```python
from build123d import *

# Parameters (mm, degrees)
SKETCH1_R                                        = 1.27
BOSS_EXTRUDE1_DEPTH                              = 25.4
CSK_FOR_1_4_FLAT_HEAD_MACHINE_SCREW1_D           = 6.7564
CSK_FOR_1_4_FLAT_HEAD_MACHINE_SCREW1_CSINK_D     = 13.3194044
CSK_FOR_1_4_FLAT_HEAD_MACHINE_SCREW1_CSINK_ANGLE = 82
SKETCH4_R                                        = 1.016
CUT_EXTRUDE1_DEPTH                               = 40.37
SKETCH5_W                                        = 65.738203623
SKETCH5_H                                        = 8.173238607
CUT_EXTRUDE2_DEPTH                               = 40.37
FILLET1_R                                        = 0.762
SKETCH8_W                                        = 13.691843982
SKETCH8_H                                        = 25.635792988
SKETCH8_W_2                                      = 17.381844488
SKETCH8_H_2                                      = 26.703951029
CUT_EXTRUDE3_DEPTH                               = 22.082
SKETCH9_R                                        = 5.08
CUT_EXTRUDE4_DEPTH                               = 11.557
CHAMFER1_SIZE                                    = 0.762
SKETCH10_W                                       = 31.402844339
SKETCH10_H                                       = 33.249058222
SKETCH10_W_2                                     = 26.204679654
SKETCH10_H_2                                     = 29.468553059
CUT_EXTRUDE5_DEPTH                               = 2.54
SKETCH11_W                                       = 51.569967854
SKETCH11_H                                       = 49.340439169
CUT_EXTRUDE6_DEPTH                               = 22.082
FILLET3_R                                        = 2.54


with BuildPart() as part:
    # Sketch1 → Boss-Extrude1 (new body)
    with BuildSketch(Plane.XY):
        Polygon((-5.842, 18.669), (-5.842, -1.651), (-28.575, -1.651), (-28.575, -20.701), (28.575, -20.701), (28.575, -1.651), (5.842, -1.651), (5.842, 18.669), align=None)
        with Locations((14.2875, -11.176)):
            Circle(SKETCH1_R, mode=Mode.SUBTRACT)
        with Locations((-14.2875, -11.176)):
            Circle(SKETCH1_R, mode=Mode.SUBTRACT)
    extrude(amount=BOSS_EXTRUDE1_DEPTH)

    # CSK for 1/4 Flat Head Machine Screw1 (through all)
    with Locations(Plane.XY.offset(25.4)):
        with Locations((-14.2875, -11.176), (14.2875, -11.176)):
            CounterSinkHole(CSK_FOR_1_4_FLAT_HEAD_MACHINE_SCREW1_D / 2, CSK_FOR_1_4_FLAT_HEAD_MACHINE_SCREW1_CSINK_D / 2, counter_sink_angle=CSK_FOR_1_4_FLAT_HEAD_MACHINE_SCREW1_CSINK_ANGLE)

    # Sketch4 → Cut-Extrude1 (cut, through all)
    with BuildSketch(Plane(origin=(0, 18.669, 0), x_dir=(1, 0, 0), z_dir=(0, 1, 0))):
        with Locations(Location((0, -5.334, 0), (0, 0, 270))):  # turned: the seam where the file's is
            Circle(SKETCH4_R)
        with Locations(Location((0, -15.494, 0), (0, 0, 90))):  # turned: the seam where the file's is
            Circle(SKETCH4_R)
    extrude(amount=-CUT_EXTRUDE1_DEPTH, mode=Mode.SUBTRACT)

    # Sketch5 → Cut-Extrude2 (cut, through all)
    with BuildSketch(Plane(origin=(0, 18.669, 0), x_dir=(1, 0, 0), z_dir=(0, 1, 0))):
        with Locations((0.634161588, -25.168619304)):
            Rectangle(SKETCH5_W, SKETCH5_H)
    extrude(amount=-CUT_EXTRUDE2_DEPTH, mode=Mode.SUBTRACT)

    # Fillet1
    fillet1_edges = [part.edges().sort_by_distance(p)[0] for p in [
        (-5.842, 18.669, 10.541),
        (5.842, 18.669, 10.541),
    ]]
    fillet(fillet1_edges, radius=FILLET1_R)

    # Sketch8 → Cut-Extrude3 (cut, through all)
    with BuildSketch(Plane.XY.offset(21.082)):
        with Locations((30.340921991, -12.055237245)):
            Rectangle(SKETCH8_W, SKETCH8_H)
        with Locations((-32.185922244, -9.773263248)):
            Rectangle(SKETCH8_W_2, SKETCH8_H_2)
    extrude(amount=-CUT_EXTRUDE3_DEPTH, mode=Mode.SUBTRACT)

    # Sketch9 → Cut-Extrude4 (cut)
    with BuildSketch(Plane.XY.offset(21.082)):
        with Locations((14.2875, -11.176)):
            Circle(SKETCH9_R)
        with Locations((-14.2875, -11.176)):
            Circle(SKETCH9_R)
    extrude(amount=-CUT_EXTRUDE4_DEPTH, mode=Mode.SUBTRACT)

    # Chamfer1
    chamfer1_edges = [part.edges().sort_by_distance(p)[0] for p in [
        (9.2075, -11.176, 21.082),
        (-19.3675, -11.176, 21.082),
        (0, -20.701, 4.318),
        (0, -20.701, 16.51),
    ]]
    chamfer(chamfer1_edges, length=CHAMFER1_SIZE)

    # Sketch10 → Cut-Extrude5 (cut)
    with BuildSketch(Plane(origin=(0, -1.651, 0), x_dir=(1, 0, 0), z_dir=(0, 1, 0))):
        with Locations((-21.54342217, -13.037102767)):
            Rectangle(SKETCH10_W, SKETCH10_H)
        with Locations((18.944339827, -12.019274454)):
            Rectangle(SKETCH10_W_2, SKETCH10_H_2)
    extrude(amount=-CUT_EXTRUDE5_DEPTH, mode=Mode.SUBTRACT)

    # Sketch11 → Cut-Extrude6 (cut, through all)
    with BuildSketch(Plane.XY.offset(21.082)):
        with Locations((0.48369004, -1.756987777)):
            Rectangle(SKETCH11_W, SKETCH11_H)
        with BuildLine():
            Line((14.2875, -4.191), (5.842, -4.191))
            Line((5.842, -4.191), (5.842, 17.907))
            ThreePointArc((5.842, 17.907), (5.618815367, 18.445815367), (5.08, 18.669))
            Line((5.08, 18.669), (-5.08, 18.669))
            ThreePointArc((-5.08, 18.669), (-5.618815367, 18.445815367), (-5.842, 17.907))
            Line((-5.842, 17.907), (-5.842, -4.191))
            Line((-5.842, -4.191), (-14.2875, -4.191))
            ThreePointArc((-14.2875, -4.191), (-21.2725, -11.176), (-14.2875, -18.161))
            Line((-14.2875, -18.161), (14.2875, -18.161))
            ThreePointArc((14.2875, -18.161), (21.2725, -11.176), (14.2875, -4.191))
        make_face(mode=Mode.SUBTRACT)
    extrude(amount=-CUT_EXTRUDE6_DEPTH, mode=Mode.SUBTRACT)

    # Fillet3
    fillet3_edges = [part.edges().sort_by_distance(p)[0] for p in [
        (-5.842, -4.191, 10.541),
        (5.842, -4.191, 10.541),
    ]]
    fillet(fillet3_edges, radius=FILLET3_R)


solid = part.part
```
Could you check a few things on this model? Use its own coordinates, in mm. A direction names the side the tool comes from. Round coordinates to 2 decimals unless told otherwise and drop trailing zeros. Write each loop counter-clockwise with the first axis right and the second up, starting at its lowest first coordinate (ties: lowest second). Pieces come first, ordered by that corner, then holes. Notation, with made-up numbers: M 12,84.5 L 38,84.5 A21 cw 38,105.5 Z; hole C 82,29 d11. An arc over 180 degrees is marked long. Answer in a Markdown table with one row per item. Add a question column.
Q1. On a 3-axis mill with a long thin cutter (end or side, diameter ignored), from which of +Z, -Z, +X, -X, +Y, -Y can I reach the whole of each face in a straight line? I mean faces 5 (the cylindrical face through (13.186, -16.135, 14.998)), 6 (the flat face through (-11, -4.191, 10)), 7 (the flat face through (5.842, 8, 10)), 8 (the cylindrical face through (-0.04, 0.51, 16.51)). Say none if no direction works.
Q2. Imagine slicing it at C-C (z = 5.75). Please give me the cut outline in (x, y) (1 decimal), then the cut area to 3 significant figures.
Q3. If I drill on line 1 (X direction, y = -13, z = 8); line 2 (X direction, y = -10, z = 6); line 3 (X direction, y = -15.5, z = 18), over which ranges is the centre line in solid material (lowest first)? Write a range as from..to.
Q4. Imagine slicing it at A-A (z = 16). Please give me the cut outline in (x, y) (1 decimal), then the cut area to 3 significant figures.
Q5. If we mould it in two halves opening along X, with no side actions, what happens to faces 1 (the cylindrical face through (0.31, 0.51, 6.3)), 2 (the cylindrical face through (6.57, -3.43, 10.39)), 3 (the cylindrical face through (17.662, -11.027, 4.696)), 4 (the cylindrical face through (-6.61, -3.47, 10.39))? For each: +X half, -X half, draft (parallel to the pull), parting line (faces both ways), or undercut.
Q6. Imagine slicing it at B-B (x = 0). Please give me the cut outline in (y, z), then the cut area to 3 significant figures.
Q7. Will these pins go through, and if not, where does the flat tip stop? pin 1 Ø6.5 at (x, z) = (-12, 14.5) entering from +Y; pin 2 Ø2 at (y, z) = (10, 8.5) entering from -X; pin 3 Ø3 at (y, z) = (-4, 17) entering from +X; pin 4 Ø1.5 at (x, y) = (-5, -8) entering from -Z.
Q8. Imagine slicing it at D-D (y = 10). Please give me the cut outline in (x, z).
Values:
| question | item | result |
|---|---|---|
| 1 | face 5 | +Z |
| 1 | face 6 | +Z, -Z, -X, +Y |
| 1 | face 7 | +Z, -Z, +X, +Y |
| 1 | face 8 | +Y, -Y |
| 2 | outline | M -14.3,-18.2 L -0.9,-18.2 L -0.9,18.7 L -5.1,18.7 A0.8 ccw -5.8,17.9 L -5.8,-1.7 A2.5 cw -8.4,-4.2 L -14.3,-4.2 A7 ccw Z; M 0.9,-18.2 L 14.3,-18.2 A7 ccw 14.3,-4.2 L 8.4,-4.2 A2.5 cw 5.8,-1.7 L 5.8,17.9 A0.8 ccw 5.1,18.7 L 0.9,18.7 Z; hole C -14.3,-11.2 d6.8; hole C 14.3,-11.2 d6.8 |
| 2 | area | 682 mm^2 |
| 3 | line 1 | -21.03..-17.13, -11.44..11.44, 17.13..21.03 |
| 3 | line 2 | -21.17..-17.45, -11.12..-0.77, 0.77..11.12, 17.45..21.17 |
| 3 | line 3 | -19.77..-16.95, -11.62..11.62, 16.95..19.77 |
| 4 | outline | M -14.3,-18.2 L -0.9,-18.2 L -0.9,18.7 L -5.1,18.7 A0.8 ccw -5.8,17.9 L -5.8,-1.7 A2.5 cw -8.4,-4.2 L -14.3,-4.2 A7 ccw Z; M 0.9,-18.2 L 14.3,-18.2 A7 ccw 14.3,-4.2 L 8.4,-4.2 A2.5 cw 5.8,-1.7 L 5.8,17.9 A0.8 ccw 5.1,18.7 L 0.9,18.7 Z; hole C -14.3,-11.2 d10.2; hole C 14.3,-11.2 d10.2 |
| 4 | area | 595 mm^2 |
| 5 | face 1 | undercut |
| 5 | face 2 | +X half |
| 5 | face 3 | undercut |
| 5 | face 4 | -X half |
| 6 | outline | M -18.16,0 L 18.67,0 L 18.67,4.32 L -18.16,4.32 Z; M -18.16,6.35 L 18.67,6.35 L 18.67,14.48 L -18.16,14.48 Z; M -18.16,16.51 L 18.67,16.51 L 18.67,21.08 L -18.16,21.08 Z |
| 6 | area | 627 mm^2 |
| 7 | pin 1 | y = -4.19 |
| 7 | pin 2 | x = -5.84 |
| 7 | pin 3 | x = 18.36 |
| 7 | pin 4 | z = 0 |
| 8 | outline | M -5.84,0 L 5.84,0 L 5.84,21.08 L -5.84,21.08 Z; hole C 0,5.33 d2.03; hole C 0,15.49 d2.03 |
